```python
from build123d import *

# Parameters (mm, degrees)
F0_W     = 333.375
F0_H     = 457.2
F0_W_2   = 307.975
F0_H_2   = 431.8
F1_DEPTH = 101.6
F2_W     = 307.975
F2_H     = 6.35
F3_DEPTH = 431.8


with BuildPart() as f1:
    # F0 (on Top) → F1 (new body)
    with BuildSketch(Plane.XY):
        Rectangle(F0_W, F0_H)
        Rectangle(F0_W_2, F0_H_2, mode=Mode.SUBTRACT)
    extrude(amount=F1_DEPTH)

    # F2 (on face) → F3 (join)
    with BuildSketch(Plane.XZ.offset(-215.9)):
        with Locations((0, 9.525)):
            Rectangle(F2_W, F2_H)
    extrude(amount=F3_DEPTH)


solid = f1.part
```
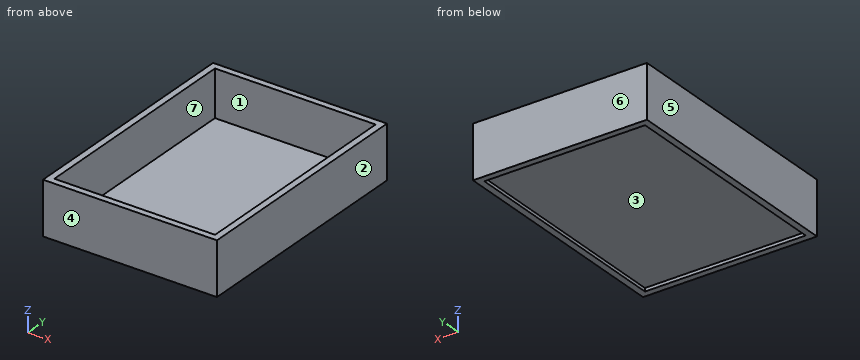
Verification items for the finished model (mm, model axes). Face numbers are marked on the shaded views. A direction names the side the tool comes from. Round coordinates to 2 decimals unless told otherwise and drop trailing zeros. Write each loop counter-clockwise with the first axis right and the second up, starting at its lowest first coordinate (ties: lowest second). Pieces come first, ordered by that corner, then holes. Notation, with made-up numbers: (6, 86.25) -> (16, 86.25) arc R16 ccw to (16, 101.25) -> close; hole circle Ø10 at (-29, -6). An arc over 180 degrees is marked (long way). Write each question's results on one line, items separated by ' | '.
Q1. Sectioned sample at C-C, the plane y = 162.5. Record the boundary of the cut face in (x, z).
Derived:
outline: (-166.69, 0) -> (-153.99, 0) -> (-153.99, 6.35) -> (153.99, 6.35) -> (153.99, 0) -> (166.69, 0) -> (166.69, 101.6) -> (153.99, 101.6) -> (153.99, 12.7) -> (-153.99, 12.7) -> (-153.99, 101.6) -> (-166.69, 101.6) -> close
Q2. Go/stop test with a flat-tipped pin: pin 1 Ø6 at (x, y) = (69.5, 54) entering from +Z. Record where the tip stops, or that it passes through.
Derived:
pin 1: stops at z = 12.7
Q3. Sectioned sample at A-A, the plane z = 92. Record the boundary of the cut face in (x, y), and give its area (3 significant figures).
Derived:
outline: (-166.69, -228.6) -> (166.69, -228.6) -> (166.69, 228.6) -> (-166.69, 228.6) -> close; hole (-153.99, -215.9) -> (153.99, -215.9) -> (153.99, 215.9) -> (-153.99, 215.9) -> close | area: 19,400 mm²
Q4. Thickness scan on probe 1 along X at (y, z) = (-209.5, 41); probe 2 along Y at (x, z) = (-29, 97.5); probe 3 along Z at (x, y) = (88.5, -188). Record the ranges inside material, lowest first.
Derived:
probe 1: x = -166.69 to -153.99, 153.99 to 166.69 | probe 2: y = -228.6 to -215.9, 215.9 to 228.6 | probe 3: z = 6.35 to 12.7
Q5. Access from +Z, -Z, +X, -X, +Y, -Y to the whole of each face (thin tool, end or side, straight path). Record for the marked faces 1, 2 and 3.
Derived:
face 1: +Z | face 2: +Z, -Z, +X, +Y, -Y | face 3: -Z
Q6. Draft check along Y on the marked faces 4, 5, 6 and 7. Enter one of: released by +Y, released by -Y, zero draft, split by the parting line, or undercut.
Derived:
face 4: released by -Y | face 5: zero draft | face 6: released by +Y | face 7: undercut
Q7. Sectioned sample at B-B, the plane x = -48. Record the boundary of the cut face in (y, z).
Derived:
outline: (-228.6, 0) -> (-215.9, 0) -> (-215.9, 6.35) -> (215.9, 6.35) -> (215.9, 0) -> (228.6, 0) -> (228.6, 101.6) -> (215.9, 101.6) -> (215.9, 12.7) -> (-215.9, 12.7) -> (-215.9, 101.6) -> (-228.6, 101.6) -> close
